CAD build for the part. Positions are in the model's coordinates, mm. Face numbers are marked on the shaded views. A direction names the side the tool comes from. Coordinates: 2 decimals unless noted, no trailing zeros. Order: outer loops, then holes, each group sorted by start corner. A loop starts at its lowest first (then second) coordinate and runs counter-clockwise, first axis right, second up. Notation, with made-up numbers: (-30, -10.5) - (28, -10.5) arc R22 ccw to (28, 13.5) - close; hole circle Ø9 at (62.25, 7). An arc over 180 degrees is marked (long way). Write each question's results on one line, items separated by ' | '. Start each with the question number.
Q1. Band-saw the part on D-D, the plane y = 33. Write the cut outline in (x, z), then the cut area to 3 significant figures.
Q2. Band-saw the part on C-C, the plane x = -11. Write the cut outline in (y, z), then the cut area to 3 significant figures.
Q3. Band-saw the part on A-A, the plane z = 11.3. Write the cut outline in (x, y).
Q4. Band-saw the part on B-B, the plane x = -17.25. Write the cut outline in (y, z), then the cut area to 3 significant figures.
Q5. Pull direction X, two halves, no side cores. Call the marked faces 1 and 2: released by +X, released by -X, zero draft, split by the parting line, or undercut.
Q6. Which spindle directions (+Z, -Z, +X, -X, +Y, -Y) get a long thin tool onto all of the face, cutting with end or side? Do the marked faces 3, 4, 5 and 6. Say none if no direction does.
Q7. Pin check, flat tips, straight feed: P1, Ø4, axis at y = 35, z = 6, coming from the -X side; P2, Ø5, axis at x = 17.25, z = 11.3, coming from the -Y side; P3, Ø7, axis at x = -3.5, y = 28, coming from the +Z side; P4, Ø1.8, axis at y = 30.5, z = 0, coming from the -X side. Stop position of each tip, or through.
Q8. Wall check: probe 1 along X at (y, z) = (62.05, 11.3); probe 2 along Y at (x, z) = (-1.5, -0.5); probe 3 along Z at (x, y) = (17.25, 61.4). Give the ranges that are in metal, low to high.
```python
from build123d import *

# Parameters (mm, degrees)
RESSALTO_EXTRUS_O1_DEPTH = 63
ESBO_O2_W                = 3.8
ESBO_O2_H                = 20
CORTE_EXTRUS_O1_DEPTH    = 41
ESBO_O3_W                = 40
ESBO_O3_H                = 2
RESSALTO_EXTRUS_O2_DEPTH = 15
ESBO_O4_R                = 1.55
CORTE_EXTRUS_O2_DEPTH    = 3
ESBO_O5_W                = 0.3
ESBO_O5_H                = 17
CORTE_EXTRUS_O3_DEPTH    = 64
ESBO_O6_W                = 3.6
ESBO_O6_H                = 2.2
CORTE_EXTRUS_O4_DEPTH    = 43
ESBO_O7_W                = 39.4
ESBO_O7_H                = 0.1
CORTE_EXTRUS_O5_DEPTH    = 46
CORTE_EXTRUS_O6_DEPTH    = 43
ESBO_O9_W                = 39.4
ESBO_O9_H                = 0.2
CORTE_EXTRUS_O7_DEPTH    = 10


with BuildPart() as part:
    # Esboço1 → Ressalto-extrusão1 (new body)
    with BuildSketch(Plane(origin=(0, 0, 0), x_dir=(1, 0, 0), z_dir=(0, 1, 0))):
        Polygon((-20, 2.9), (20, 2.9), (20, 0.9), (16.5, 0.9), (16.5, -0.9), (20, -0.9), (20, -2.9), (-20, -2.9), (-20, -0.9), (-16.5, -0.9), (-16.5, 0.9), (-20, 0.9), align=None)
    extrude(amount=RESSALTO_EXTRUS_O1_DEPTH)

    # Esboço2 → Corte-extrusão1 (cut, through all)
    with BuildSketch(Plane(origin=(20, 0, 0), x_dir=(0, 0, -1), z_dir=(1, 0, 0))):
        with Locations((-1, 53)):
            Rectangle(ESBO_O2_W, ESBO_O2_H)
    extrude(amount=-CORTE_EXTRUS_O1_DEPTH, mode=Mode.SUBTRACT)

    # Esboço3 → Ressalto-extrusão2 (add)
    with BuildSketch(Plane.XY.offset(-0.9)):
        with Locations((0, 62)):
            Rectangle(ESBO_O3_W, ESBO_O3_H)
    extrude(amount=RESSALTO_EXTRUS_O2_DEPTH)

    # Esboço4 → Corte-extrusão2 (cut)
    with BuildSketch(Plane(origin=(0, 63, 0), x_dir=(1, 0, 0), z_dir=(0, 1, 0))):
        with Locations((-17.25, -11.3)):
            Circle(ESBO_O4_R)
        with Locations((17.25, -11.3)):
            Circle(ESBO_O4_R)
    extrude(amount=-CORTE_EXTRUS_O2_DEPTH, mode=Mode.SUBTRACT)

    # Esboço5 → Corte-extrusão3 (cut, through all)
    with BuildSketch(Plane.XZ):
        with Locations((-19.85, 5.6)):
            Rectangle(ESBO_O5_W, ESBO_O5_H)
        with Locations((19.85, 5.6)):
            Rectangle(ESBO_O5_W, ESBO_O5_H)
    extrude(amount=-CORTE_EXTRUS_O3_DEPTH, mode=Mode.SUBTRACT)

    # Esboço6 → Corte-extrusão4 (cut)
    with BuildSketch(Plane.XZ):
        with Locations((18.1, 0)):
            Rectangle(ESBO_O6_W, ESBO_O6_H)
        with Locations((-18.1, 0)):
            Rectangle(ESBO_O6_W, ESBO_O6_H)
    extrude(amount=-CORTE_EXTRUS_O4_DEPTH, mode=Mode.SUBTRACT)

    # Esboço7 → Corte-extrusão5 (cut)
    with BuildSketch(Plane.XZ):
        with Locations((0, 2.85)):
            Rectangle(ESBO_O7_W, ESBO_O7_H)
    extrude(amount=-CORTE_EXTRUS_O5_DEPTH, mode=Mode.SUBTRACT)

    # Esboço8 → Corte-extrusão6 (cut)
    with BuildSketch(Plane.XZ):
        Polygon((9.7, 2.8), (6.9, 0), (-6.135691889, 0), (-6.9, 0), (-9.7, 2.8), align=None)
    extrude(amount=-CORTE_EXTRUS_O6_DEPTH, mode=Mode.SUBTRACT)

    # Esboço9 → Corte-extrusão7 (cut)
    with BuildSketch(Plane.XY.offset(2.8)):
        with Locations((0, 0.1)):
            Rectangle(ESBO_O9_W, ESBO_O9_H)
    extrude(amount=-CORTE_EXTRUS_O7_DEPTH, mode=Mode.SUBTRACT)


solid = part.part
```
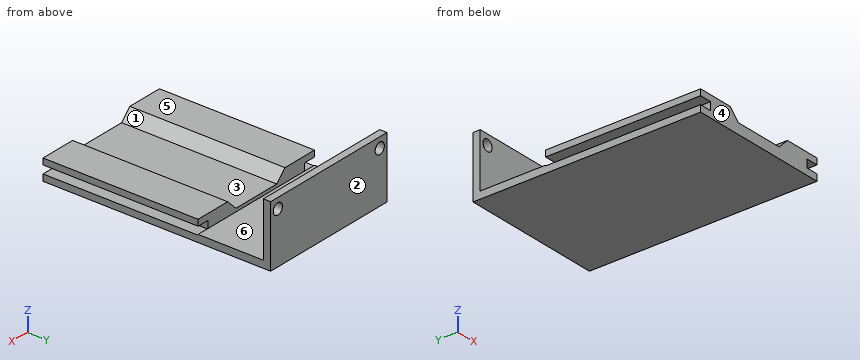
Results below:
1) outline: (-19.7, -2.9) - (19.7, -2.9) - (19.7, -1.1) - (16.3, -1.1) - (16.3, 1.1) - (19.7, 1.1) - (19.7, 2.8) - (9.7, 2.8) - (6.9, 0) - (-6.9, 0) - (-9.7, 2.8) - (-19.7, 2.8) - (-19.7, 1.1) - (-16.3, 1.1) - (-16.3, -1.1) - (-19.7, -1.1) - close | area: 163 mm²
2) outline: (0.2, -2.9) - (63, -2.9) - (63, 14.1) - (61, 14.1) - (61, -0.9) - (43, -0.9) - (43, 2.8) - (0.2, 2.8) - close | area: 314 mm²
3) outline: (-19.7, 61) - (-18.8, 61) - (-18.8, 63) - (-19.7, 63) - close; (-15.7, 61) - (15.7, 61) - (15.7, 63) - (-15.7, 63) - close; (18.8, 61) - (19.7, 61) - (19.7, 63) - (18.8, 63) - close
4) outline: (0.2, -2.9) - (63, -2.9) - (63, 9.75) - (61, 9.75) - (61, -0.9) - (43, -0.9) - (43, -1.1) - (0.2, -1.1) - close; (0.2, 1.1) - (43, 1.1) - (43, 2.8) - (0.2, 2.8) - close; (61, 12.85) - (63, 12.85) - (63, 14.1) - (61, 14.1) - close | area: 214 mm²
5) face 1: undercut | face 2: zero draft
6) face 3: +Z, -Y | face 4: +Z, -Z, +X, -X, -Y | face 5: +Z, +X, -X, -Y | face 6: +Z, +X, -X
7) P1: passes through | P2: stops at y = 61 | P3: stops at z = 0.1 | P4: stops at x = -16.3
8) probe 1: x = -19.7 to -18.8, -15.7 to 15.7, 18.8 to 19.7 | probe 2: y = 0.2 to 43, 61 to 63 | probe 3: z = -2.9 to 9.75, 12.85 to 14.1
